CAD build for the part. Positions are in the model's coordinates, mm. A direction names the side the tool comes from. Coordinates: 2 decimals unless noted, no trailing zeros. Write each loop counter-clockwise with the first axis right and the second up, starting at its lowest first coordinate (ties: lowest second). Pieces come first, ordered by that corner, then holes. Notation, with made-up numbers: M 53.5,-16.75 L 76.5,-16.75 A24 cw 76.5,9.25 Z; hole C -39,-2 d7. An arc over 180 degrees is marked long. Put each result on its own line as item: value. Start each with the question number.
```python
from build123d import *

# Parameters (mm, degrees)
F0_W     = 25.4
F0_H     = 50.8
F1_DEPTH = 146.05
F2_W     = 9.525
F2_H     = 25.4
F3_DEPTH = 3.175
F5_D     = 6.35
F5_DEPTH = 38.1
F5_TIP   = 1.9077324654
F7_D     = 6.35
F7_DEPTH = 38.1
F7_TIP   = 1.9077324654
F9_D     = 6.3754


with BuildPart() as f1:
    # F0 (on Right) → F1 (new body)
    with BuildSketch(Plane.YZ):
        with Locations((-0.2286629751, 10.6222124508)):
            Rectangle(F0_W, F0_H)
    extrude(amount=F1_DEPTH)

    # F2 (on face) → F3 (cut)
    with BuildSketch(Plane(origin=(0, 0, -14.7777875492), x_dir=(1, 0, 0), z_dir=(0, 0, -1))):
        with Locations((141.2875, 0.2286629751)):
            Rectangle(F2_W, F2_H)
        with Locations((4.7625, 0.2286629751)):
            Rectangle(F2_W, F2_H)
    extrude(amount=-F3_DEPTH, mode=Mode.SUBTRACT)

    # F5
    with Locations(Plane.YZ.offset(146.05)):
        with Locations((0, 23.3222124508), (0, -2.0777875492)):
            Hole(F5_D / 2, depth=F5_DEPTH)
            with Locations((0, 0, -(F5_DEPTH + F5_TIP / 2))):  # 118° drill point
                Cone(0, F5_D / 2, F5_TIP, mode=Mode.SUBTRACT)

    # F7
    with Locations(Plane(origin=(0, 0, 0), x_dir=(0, -1, 0), z_dir=(-1, 0, 0))):
        with Locations((0.2286629751, 23.3222124508), (0.2286629751, -2.0777875492)):
            Hole(F7_D / 2, depth=F7_DEPTH)
            with Locations((0, 0, -(F7_DEPTH + F7_TIP / 2))):  # 118° drill point
                Cone(0, F7_D / 2, F7_TIP, mode=Mode.SUBTRACT)

    # F9 (through all)
    with Locations(Plane(origin=(0, 0, -14.7777875492), x_dir=(1, 0, 0), z_dir=(0, 0, -1))):
        with Locations((123.825, -6.1213370249), (22.225, -6.1213370249)):
            Hole(F9_D / 2)


solid = f1.part
```
(1) Which spindle directions (+Z, -Z, +X, -X, +Y, -Y) get a long thin tool onto all of the face, cutting with end or side? Do faces 4 (the face through (19.317, -0.917, -5.177)), 5 (the face through (5, 0, -11.603)), 6 (the face through (136.525, 0, -13)), 7 (the face through (126.733, 0.688, -5.177)). Say none if no direction does.
(2) Drill centre lines: line 1 (X direction, y = 6, z = -10.5); line 2 (X direction, y = 5.25, z = 27.5); line 3 (Z direction, x = 23.5, y = 2.25). Where is each one in solid material? Low to high. Write a range as [from, to].
(3) Two-plate mould, pull along Y, no slides. Class faces 1 (the face through (72, 0, 36.022)), 2 (the face through (126.733, 0.688, 20.223)), 3 (the face through (72, -12.929, 10)): +Y half, -Y half, draft (parallel to the pull), parting line (faces both ways), or undercut.
(4) Drop flat-ended pins along their axis: pin 1 (7.5 mm diameter, centred on y = -0.23, z = 23.32, fed in from +X); pin 2 (4 mm diameter, centred on y = 0, z = -2.08, fed in from +X); pin 3 (7.5 mm diameter, centred on x = 143, y = -6, fed in from -Z); pin 4 (5.5 mm diameter, centred on x = 22.22, y = 6.12, fed in from -Z). Give the stop position or say it passes through.
(5) Slice it at A-A, the plane z = -7. Write the cut outline in (x, y) (3 decimals), then the cut area to 3 significant figures.
(6) Slice it at B-B, the plane x = 31. Write the cut outline in (y, z) (3 decimals), then the cut area to 3 significant figures.
Result set:
1. face 4: -X
1. face 5: -Z, -X, +Y, -Y
1. face 6: -Z, +X, +Y, -Y
1. face 7: +X
2. line 1: x = [0, 19.04], [25.41, 120.64], [127.01, 146.05]
2. line 2: x = [0, 19.16], [25.29, 120.76], [126.89, 146.05]
2. line 3: z = [-14.78, -4.06], [-0.09, 21.34], [25.31, 36.02]
3. face 1: draft
3. face 2: undercut
3. face 3: -Y half
4. pin 1: stops at x = 146.05
4. pin 2: stops at x = 107.25
4. pin 3: stops at z = -11.6
4. pin 4: passes through
5. outline: M 0,-12.929 L 146.05,-12.929 L 146.05,12.471 L 0,12.471 Z; hole C 22.225,6.121 d6.375; hole C 123.825,6.121 d6.375
5. area: 3,650 mm^2
6. outline: M -12.929,-14.778 L 12.471,-14.778 L 12.471,36.022 L -12.929,36.022 Z; hole C -0.229,-2.078 d6.35; hole C -0.229,23.322 d6.35
6. area: 1,230 mm^2
